Geometry check sheet. Reference: the model listing, model coordinates, mm. Face numbers are marked on the shaded views. A direction names the side the tool comes from. Round coordinates to 2 decimals unless told otherwise and drop trailing zeros. Write each loop counter-clockwise with the first axis right and the second up, starting at its lowest first coordinate (ties: lowest second). Pieces come first, ordered by that corner, then holes. Notation, with made-up numbers: M -10,71.5 L -3,71.5 A13 ccw -3,89.5 Z; hole C 40,-17.5 d4. An arc over 180 degrees is marked long. One line per item, written item: value. Start each with the question number.
1. Release check for a two-part mould opening along Y. For the marked faces 1, 2 and 3 record: pulls with the +Y half, pulls with the -Y half, needs draft (parallel to the pull), parting line crosses it, or undercut.
2. Section check D-D (x = 2.25). Record the boundary of the cut face in (y, z) (3 decimals).
3. Section check B-B (x = 4.5). Record the boundary of the cut face in (y, z) (3 decimals), and give its area (3 significant figures).
4. Section check A-A (z = 4.75). Record the boundary of the cut face in (x, y) (3 decimals).
5. Scan lines: probe 1 along X at (y, z) = (-3, 8.5) (3 decimals); probe 2 along Z at (x, y) = (11, 1.25) (3 decimals); probe 3 along Z at (x, y) = (8.75, -2.25) (3 decimals). Record each from-to range of solid material in increasing order. Write a range as [from, to].
6. Section check C-C (y = 0). Count the separate pieces of the cut face and the enclosed holes in it, and give its area (3 significant figures).
7. Access from +Z, -Z, +X, -X, +Y, -Y to the whole of each face (thin tool, end or side, straight path). Record for the marked faces 4, 5, 6, 7 and 8.
8. Depth check by flat-ended pin: P1, Ø2, axis at x = 13.5, z = 6, coming from the +Y side; P2, Ø6, axis at x = 9, z = 14, coming from the -Y side; P3, Ø3, axis at x = 5, z = 18.5, coming from the -Y side. Enter the tip coordinate at first touch or a pass-through.
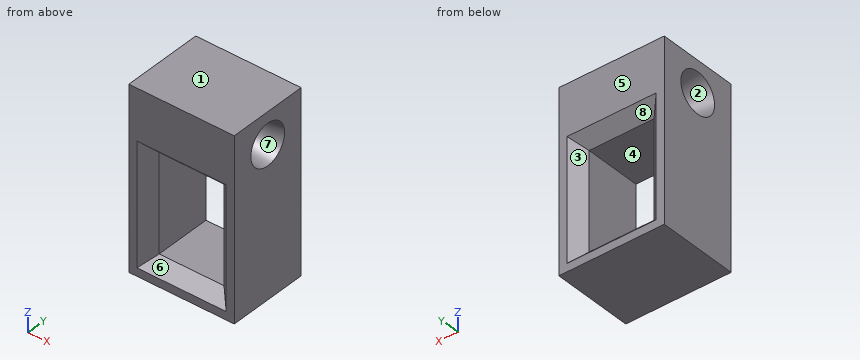
from build123d import *

# Parameters (mm, degrees)
F0_W     = 16.51
F0_H     = 28.265
F0_W_2   = 10.16
F0_H_2   = 15.24
F1_DEPTH = 6.35
F2_SIZE  = 1.905
F4_R     = 1.75
F5_DEPTH = 12.7
F5_TAPER = -10
F6_R     = 12.7


with BuildPart() as f1:
    # F0 (on Front) → F1 (new body, symmetric)
    with BuildSketch(Plane.XZ):
        with Locations((8.255, 14.1325)):
            Rectangle(F0_W, F0_H)
        with Locations((8.255, 10.795)):
            Rectangle(F0_W_2, F0_H_2, mode=Mode.SUBTRACT)
    extrude(amount=F1_DEPTH, both=True)

    # F2
    f2_edges = [f1.edges().sort_by_distance(p)[0] for p in [
        (13.335, -6.35, 10.795),
        (8.255, -6.35, 18.415),
        (3.175, -6.35, 10.795),
        (8.255, -6.35, 3.175),
        (3.175, 6.35, 10.795),
        (8.255, 6.35, 18.415),
        (8.255, 6.35, 3.175),
        (13.335, 6.35, 10.795),
    ]]
    chamfer(f2_edges, length=F2_SIZE)

    # F4 (on mid) → F5 (cut, symmetric)
    with BuildSketch(Plane(origin=(8.255, 0, 0), x_dir=(0, -1, 0), z_dir=(-1, 0, 0))):
        with Locations((0, 23.34)):
            Circle(F4_R)
    extrude(amount=F5_DEPTH, both=True, taper=F5_TAPER, mode=Mode.SUBTRACT)

    # F6
    f6_edges = [f1.edges().sort_by_distance(p)[0] for p in [
        (8.255, 1.75, 23.34),
    ]]
    fillet(f6_edges, radius=F6_R)


solid = f1.part
Result sheet:
1. face 1: needs draft
1. face 2: undercut
1. face 3: pulls with the +Y half
2. outline: M -6.35,0 L 6.35,0 L 6.35,1.27 L 5.37,2.25 L 5.37,19.34 L 6.35,20.32 L 6.35,28.265 L -6.35,28.265 L -6.35,20.32 L -5.37,19.34 L -5.37,2.25 L -6.35,1.27 Z; hole C 0,23.34 d5.618
3. outline: M -6.35,0 L 6.35,0 L 6.35,1.27 L 4.445,3.175 L -4.445,3.175 L -6.35,1.27 Z; M -6.35,20.32 L -4.445,18.415 L 4.445,18.415 L 6.35,20.32 L 6.35,28.265 L -6.35,28.265 Z; hole C 0,23.34 d4.824
3. area: 140 mm2
4. outline: M 0,-6.35 L 1.27,-6.35 L 3.175,-4.445 L 3.175,4.445 L 1.27,6.35 L 0,6.35 Z; M 13.335,-4.445 L 15.24,-6.35 L 16.51,-6.35 L 16.51,6.35 L 15.24,6.35 L 13.335,4.445 Z
5. probe 1: x = [0, 3.175], [13.335, 16.51]
5. probe 2: z = [0, 3.175], [18.415, 21.488], [25.192, 28.265]
5. probe 3: z = [0, 3.175], [18.415, 28.265]
6. separate pieces: 2
6. enclosed holes: 1
6. area: 229 mm2
7. face 4: +Y, -Y
7. face 5: +Z, -Z, +X, -X, +Y
7. face 6: -Y
7. face 7: +X
7. face 8: +Y
8. P1: stops at y = 5.61
8. P2: passes through
8. P3: stops at y = -6.03
